The drawing under review shows one solid part. Ordinate dimensions are in mm from its lowest x, y, z. Coordinates: 2 decimals unless noted, no trailing zeros. Loops run counter-clockwise (first coordinate to the right, second up) from the corner with the lowest first, then second, coordinate; pieces in that order, holes last.
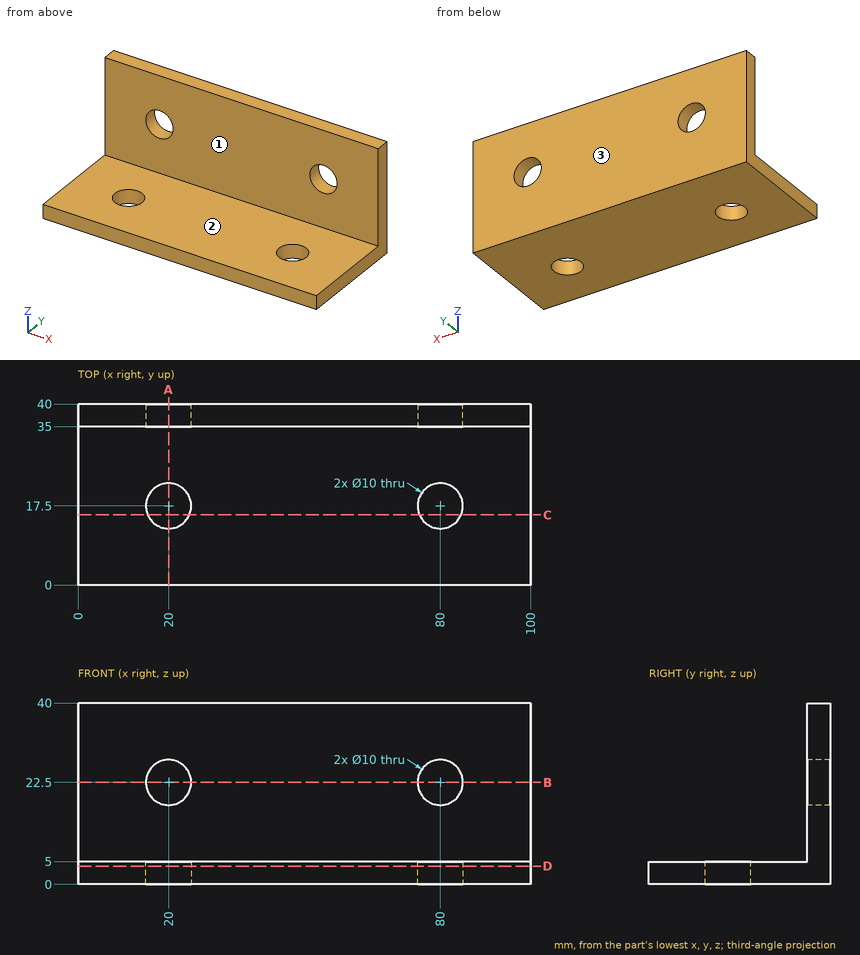
Q1. Take a section at D-D, the plane z = 4. Write out the cut boundary in (x, y), then the cut area to 3 significant figures.
Q2. For line 1 (Z direction, x = 80, y = 36.7); line 2 (X direction, y = 15, z = 2); line 3 (Z direction, x = 72.5, y = 31), list the stretches that pass through material, from the lowest coordinate up.
Q3. Clearance check with flat-ended pins moving along their axes: pin 1 Ø11.5 at (x, z) = (80, 22.5) entering from -Y; pin 2 Ø1.5 at (x, y) = (64, 29) entering from +Z; pin 3 Ø9 at (x, z) = (20, 22.5) entering from -Y. State where each tip first meets the part, or that it passes through.
Q4. Take a section at C-C, the plane y = 15.5. Write out the cut boundary in (x, z).
Q5. Take a section at A-A, the plane x = 20. Write out the cut boundary in (y, z).
Q6. The part is to be moulded in two halves that separate along Y. For the marked faces 1, 2 and 3, say which applies: pulls with the +Y half, pulls with the -Y half, needs draft (parallel to the pull), parting line crosses it, or undercut.
Q7. Take a section at B-B, the plane z = 22.5. Write out the cut boundary in (x, y), then the cut area to 3 significant figures.
Entries:
1. outline: (0, 0) - (100, 0) - (100, 40) - (0, 40) - close; hole circle Ø10 at (20, 17.5); hole circle Ø10 at (80, 17.5)
1. area: 3,840 mm2
2. line 1: z = 0 to 17.5, 27.5 to 40
2. line 2: x = 0 to 15.67, 24.33 to 75.67, 84.33 to 100
2. line 3: z = 0 to 5
3. pin 1: stops at y = 35
3. pin 2: stops at z = 5
3. pin 3: passes through
4. outline: (0, 0) - (15.42, 0) - (15.42, 5) - (0, 5) - close; (24.58, 0) - (75.42, 0) - (75.42, 5) - (24.58, 5) - close; (84.58, 0) - (100, 0) - (100, 5) - (84.58, 5) - close
5. outline: (0, 0) - (12.5, 0) - (12.5, 5) - (0, 5) - close; (22.5, 0) - (40, 0) - (40, 17.5) - (35, 17.5) - (35, 5) - (22.5, 5) - close; (35, 27.5) - (40, 27.5) - (40, 40) - (35, 40) - close
6. face 1: pulls with the -Y half
6. face 2: needs draft
6. face 3: pulls with the +Y half
7. outline: (0, 35) - (15, 35) - (15, 40) - (0, 40) - close; (25, 35) - (75, 35) - (75, 40) - (25, 40) - close; (85, 35) - (100, 35) - (100, 40) - (85, 40) - close
7. area: 400 mm2
